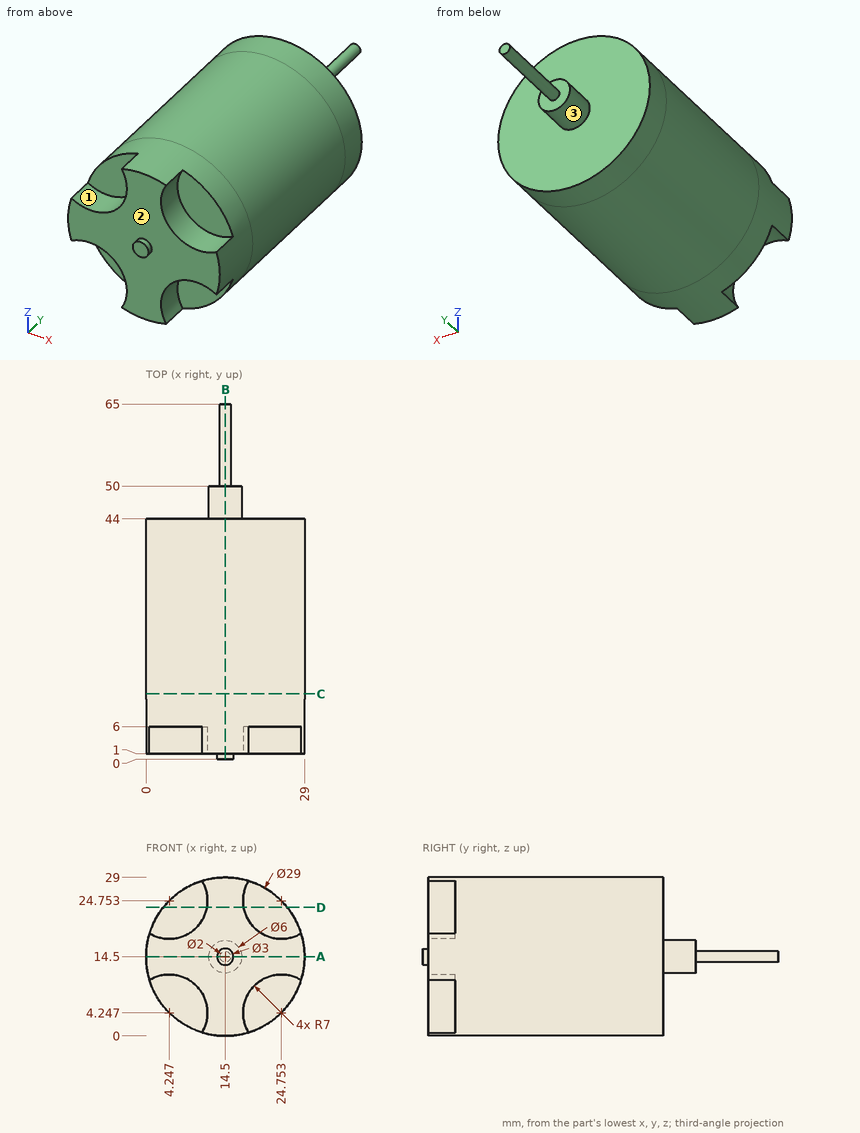
Answer from the drawing. Dimensions are ordinates in mm from the lowest x, y and z of the part. Round coordinates to 2 decimals unless told otherwise and drop trailing zeros. Write each loop counter-clockwise with the first axis right and the second up, starting at its lowest first coordinate (ties: lowest second). Pieces come first, ordered by that corner, then holes. Notation, with made-up numbers: (17.25, -34) -> (35.25, -34) arc R28 cw to (35.25, -10) -> close; hole circle Ø3 at (1.25, -25.5). An arc over 180 degrees is marked (long way). Answer in a Markdown table with one row per item. Add a question column.
1) Given P1, Ø8.5, axis at x = 24, z = 23, coming from the -Y side; P2, Ø1.5, axis at x = 17.5, z = 4.5, coming from the -Y side; P3, Ø12, axis at x = 17, z = 3.5, coming from the +Y side, each flat-ended and moving along its own axis, determine where each tip first touches the part or whether it passes through.
2) Determine the mould class of the marked faces 1, 2 and 3 for opening direction Z: pulls with the +Z half, pulls with the -Z half, needs draft (parallel to the pull), parting line crosses it, or undercut.
3) Find section C-C, the plane y = 12. Determine the outline of the cut face in (x, z), and give its area (3 significant figures).
4) Find section B-B, the plane x = 14.5. Determine the outline of the cut face in (y, z).
5) Find section D-D, the plane z = 23.5. Determine the outline of the cut face in (x, y).
6) Consider line 1 (X direction, y = 8.5, z = 15); line 2 (Z direction, x = 14.5, y = 57); line 3 (Y direction, x = 13.5, z = 13). Determine where each line is inside the solid, lowest interval first.
7) Find section A-A, the plane z = 14.5. Determine the outline of the cut face in (x, y), and give its area (3 significant figures).
Findings below:
| question | item | result |
|---|---|---|
| 1 | P1 | y = 6 |
| 1 | P2 | y = 1 |
| 1 | P3 | y = 44 |
| 2 | face 1 | undercut |
| 2 | face 2 | needs draft |
| 2 | face 3 | parting line crosses it |
| 3 | outline | circle Ø29 at (14.5, 14.5) |
| 3 | area | 661 mm² |
| 4 | outline | (0, 13) -> (1, 13) -> (1, 0) -> (44, 0) -> (44, 11.5) -> (50, 11.5) -> (50, 13.5) -> (65, 13.5) -> (65, 15.5) -> (50, 15.5) -> (50, 17.5) -> (44, 17.5) -> (44, 29) -> (1, 29) -> (1, 16) -> (0, 16) -> close |
| 5 | outline | (3.13, 6) -> (11.13, 6) -> (11.13, 1) -> (17.87, 1) -> (17.87, 6) -> (25.87, 6) -> (25.87, 44) -> (3.13, 44) -> close |
| 6 | line 1 | 0.01 to 28.99 |
| 6 | line 2 | 13.5 to 15.5 |
| 6 | line 3 | 1 to 50 |
| 7 | outline | (0, 1) -> (13, 1) -> (13, 0) -> (16, 0) -> (16, 1) -> (29, 1) -> (29, 44) -> (17.5, 44) -> (17.5, 50) -> (15.5, 50) -> (15.5, 65) -> (13.5, 65) -> (13.5, 50) -> (11.5, 50) -> (11.5, 44) -> (0, 44) -> close |
| 7 | area | 1,320 mm² |
